from build123d import *

# Parameters (mm, degrees)
SKETCH1_W           = 237
SKETCH1_H           = 56
BOSS_EXTRUDE1_DEPTH = 4
SKETCH2_R           = 2
CUT_EXTRUDE1_DEPTH  = 5
SKETCH5_W           = 30
SKETCH5_H           = 4.1
BOSS_EXTRUDE2_DEPTH = 15
SKETCH6_W           = 4
SKETCH6_H           = 56
BOSS_EXTRUDE3_DEPTH = 25
FILLET1_START       = -119
FILLET1_DEPTH       = 238
FILLET3_R           = 4
FILLET4_R           = 4
FILLET5_R           = 4
FILLET6_R           = 4


with BuildPart() as part:
    # Sketch1 → Boss-Extrude1 (new body)
    with BuildSketch(Plane(origin=(0, 0, 0), x_dir=(1, 0, 0), z_dir=(0, 1, 0))):
        Rectangle(SKETCH1_W, SKETCH1_H)
    extrude(amount=BOSS_EXTRUDE1_DEPTH)

    # Sketch2 → Cut-Extrude1 (cut)
    with BuildSketch(Plane.XZ):
        with Locations(Location((108.5, 17.5, 0), (0, 0, 270))):
            Circle(SKETCH2_R)
        with Locations(Location((108.5, -17.5, 0), (0, 0, 270))):
            Circle(SKETCH2_R)
        with Locations(Location((-108.5, -17.5, 0), (0, 0, 270))):
            Circle(SKETCH2_R)
        with Locations(Location((-108.5, 17.5, 0), (0, 0, 270))):
            Circle(SKETCH2_R)
    extrude(amount=-CUT_EXTRUDE1_DEPTH, mode=Mode.SUBTRACT)

    # Sketch5 → Boss-Extrude2 (add)
    with BuildSketch(Plane(origin=(0, 4, 0), x_dir=(1, 0, 0), z_dir=(0, 1, 0))):
        with Locations((0, -25.95)):
            Rectangle(SKETCH5_W, SKETCH5_H)
        with Locations((25, 25.95)):
            Rectangle(SKETCH5_W, SKETCH5_H)
        with Locations((-25, 25.95)):
            Rectangle(SKETCH5_W, SKETCH5_H)
    extrude(amount=BOSS_EXTRUDE2_DEPTH)

    # Sketch6 → Boss-Extrude3 (add)
    with BuildSketch(Plane(origin=(0, 4, 0), x_dir=(1, 0, 0), z_dir=(0, 1, 0))):
        with Locations((-97.5, 0)):
            Rectangle(SKETCH6_W, SKETCH6_H)
        with Locations((97.5, 0)):
            Rectangle(SKETCH6_W, SKETCH6_H)
    extrude(amount=BOSS_EXTRUDE3_DEPTH)

    # Fillet1: read off the stored shape, not the designer's step
    # Fillet1 outline → Fillet1 (cut)
    with BuildSketch(Plane.YZ.offset(FILLET1_START)):
        with BuildLine():
            ThreePointArc((4, -28), (1.171572875, -26.828427125), (0, -24))
            Line((0, -24), (0, -28))
            Line((0, -28), (4, -28))
        make_face()
    extrude(amount=FILLET1_DEPTH, mode=Mode.SUBTRACT)

    # Fillet3
    fillet3_edges = [part.edges().sort_by_distance(p)[0] for p in [
        (0, 4, 23.9),
        (25, 4, -23.9),
        (-25, 4, -23.9),
        (-95.5, 4, 0),
        (95.5, 4, 0),
    ]]
    fillet(fillet3_edges, radius=FILLET3_R)

    # Fillet4
    # the kernel refuses this fillet: 4 mm, written as the material it takes off along each edge
    with BuildSketch(Plane(origin=(-118.5, 4, -38), x_dir=(0, -1, 0), z_dir=(0, 0, 1)), Plane(origin=(-99.5, 29, -38), x_dir=(0, -1, 0), z_dir=(0, 0, 1))) as fillet4_piece_1:
        with BuildLine():
            CenterArc((FILLET4_R, FILLET4_R), FILLET4_R, 180, 90)
            Line((0, FILLET4_R), (0, 0))
            Line((0, 0), (FILLET4_R, 0))
        make_face()
    extrude(amount=76, mode=Mode.SUBTRACT)
    with BuildSketch(Plane(origin=(118.5, 4, 38), x_dir=(-1, 0, 0), z_dir=(0, 0, -1)), Plane(origin=(99.5, 29, 38), x_dir=(-1, 0, 0), z_dir=(0, 0, -1))) as fillet4_piece_2:
        with BuildLine():
            CenterArc((FILLET4_R, -FILLET4_R), FILLET4_R, 90, 90)
            Line((0, -FILLET4_R), (0, 0))
            Line((0, 0), (FILLET4_R, 0))
        make_face()
    extrude(amount=76, mode=Mode.SUBTRACT)
    with BuildSketch(Plane(origin=(-99.5, 4, -28), x_dir=(1, 0, 0), z_dir=(0, 1, 0)), Plane(origin=(99.5, 4, 28), x_dir=(-1, 0, 0), z_dir=(0, 1, 0))) as fillet4_piece_3:
        with BuildLine():
            CenterArc((FILLET4_R, -FILLET4_R), FILLET4_R, 90, 90)
            Line((0, -FILLET4_R), (0, 0))
            Line((0, 0), (FILLET4_R, 0))
        make_face()
    extrude(amount=35, mode=Mode.SUBTRACT)
    with BuildSketch(Plane(origin=(-99.5, 4, 28), x_dir=(1, 0, 0), z_dir=(0, 1, 0)), Plane(origin=(99.5, 4, -28), x_dir=(-1, 0, 0), z_dir=(0, 1, 0))) as fillet4_piece_4:
        with BuildLine():
            CenterArc((FILLET4_R, FILLET4_R), FILLET4_R, 180, 90)
            Line((0, FILLET4_R), (0, 0))
            Line((0, 0), (FILLET4_R, 0))
        make_face()
    extrude(amount=35, mode=Mode.SUBTRACT)

    # Fillet5
    fillet5_edges = [part.edges().sort_by_distance(p)[0] for p in [
        (15, 11.5, 28),
        (-15, 11.5, 28),
        (0, 19, 28),
    ]]
    fillet(fillet5_edges, radius=FILLET5_R)

    # Fillet6
    fillet6_edges = [part.edges().sort_by_distance(p)[0] for p in [
        (25, 19, -28),
        (-25, 19, -28),
    ]]
    fillet(fillet6_edges, radius=FILLET6_R)


solid = part.part
Here's how the part is built. I have some questions about the finished solid (model axes, mm). A direction names the side the tool comes from. Round coordinates to 2 decimals unless told otherwise and drop trailing zeros. Order: outer loops, then holes, each group sorted by start corner. A loop starts at its lowest first (then second) coordinate and runs counter-clockwise, first axis right, second up. Notation, with made-up numbers: (48.25, 86.25) -> (105.25, 86.25) arc R31 ccw to (105.25, 118.25) -> close; hole circle Ø2 at (88, 42.25). An arc over 180 degrees is marked (long way). Use CSV: the item, a comma, the result in double quotes.
1. Thinking about a two-plate mould opening in X: for faces 1 (the face through (-117.297, 2.859, -0.392)), 2 (the face through (-24.79, 17.797, -26.859)), 3 (the face through (-1.659, 1.203, -26.859)), which applies, pulls with the +X half, pulls with the -X half, needs draft (parallel to the pull), parting line crosses it, or undercut?
Recorded:
face 1,"pulls with the -X half"
face 2,"undercut"
face 3,"needs draft"
2. I'm going to push flat-ended pins straight in: P1, Ø9, axis at x = -2, y = 16, coming from the -Z side; P2, Ø17, axis at y = 10, z = -3.5, coming from the -X side; P3, Ø5, axis at y = 12, z = 12.5, coming from the -X side; P4, Ø5, axis at x = -58, z = -4.5, coming from the -Y side. Where does each tip first touch, or does it pass through?
Recorded:
P1,"stops at z = 23.9"
P2,"stops at x = -118.21"
P3,"stops at x = -99.5"
P4,"stops at y = 0"
3. Which directions (+Z, -Z, +X, -X, +Y, -Y) give clear straight access to the entire face, cutting with the end or side of a thin tool? Please do faces 4 (the face through (10, 10, -26)), 5 (the face through (40, 10, -26)), 6 (the face through (-15, 6.5, 23.8)), 7 (the face through (-98.297, 16.325, -26.859)), 8 (the face through (-98.359, 16.325, 26.797)).
Recorded:
face 4,"-Z, +Y"
face 5,"+Z, -Z, +Y"
face 6,"+Z, +Y"
face 7,"-Z, -X, +Y"
face 8,"+Z, -X, +Y"
4. I want a section at C-C on x = -28. List the corners of the cut face in (y, z) for me.
Recorded:
outline,"(0, -24) arc R4 ccw to (4, -28) -> (15, -28) arc R4 ccw to (19, -24) -> (19, -23.9) -> (8, -23.9) arc R4 cw to (4, -19.9) -> (4, 28) -> (0, 28) -> close"
5. I want a section at D-D on z = -4.5. List the corners of the cut face in (x, y) for me.
Recorded:
outline,"(-118.5, 0) -> (118.5, 0) arc R4 ccw to (114.5, 4) -> (99.5, 4) -> (99.5, 25) arc R4 ccw to (95.5, 29) -> (95.5, 8) arc R4 cw to (91.5, 4) -> (-91.5, 4) arc R4 cw to (-95.5, 8) -> (-95.5, 29) arc R4 ccw to (-99.5, 25) -> (-99.5, 4) -> (-114.5, 4) arc R4 ccw to start"
6. I want a section at B-B on z = -17.5. List the corners of the cut face in (x, y) for me, and give its area (3 significant figures).
Recorded:
outline,"(-118.5, 0) -> (-110.5, 0) -> (-110.5, 4) -> (-114.5, 4) arc R4 ccw to start; (-106.5, 0) -> (106.5, 0) -> (106.5, 4) -> (99.5, 4) -> (99.5, 25) arc R4 ccw to (95.5, 29) -> (95.5, 8) arc R4 cw to (91.5, 4) -> (-91.5, 4) arc R4 cw to (-95.5, 8) -> (-95.5, 29) arc R4 ccw to (-99.5, 25) -> (-99.5, 4) -> (-106.5, 4) -> close; (110.5, 0) -> (118.5, 0) arc R4 ccw to (114.5, 4) -> (110.5, 4) -> close"
area,"1,110 mm2"
7. I want a section at A-A on y = 11.5. List the corners of the cut face in (x, z) for me, and give its area (3 significant figures).
Recorded:
outline,"(-99.5, -24) arc R4 ccw to (-95.5, -28) -> (-95.5, 28) arc R4 ccw to (-99.5, 24) -> close; (-40, -28) -> (-10, -28) -> (-10, -23.9) -> (-40, -23.9) -> close; (-15, 23.9) -> (15, 23.9) -> (15, 24) arc R4 ccw to (11, 28) -> (-11, 28) arc R4 ccw to (-15, 24) -> close; (10, -28) -> (40, -28) -> (40, -23.9) -> (10, -23.9) -> close; (95.5, -28) arc R4 ccw to (99.5, -24) -> (99.5, 24) arc R4 ccw to (95.5, 28) -> close"
area,"796 mm2"
8. I need wall thicknesses on line 1 along X through (y, z) = (14, -24); line 2 along X through (y, z) = (8.75, 15.5); line 3 along Y through (x, z) = (-23, 13.5). Which ranges of each line are inside material? Lowest first, please.
Recorded:
line 1,"x = -99.5 to -95.5, -40 to -10, 10 to 40, 95.5 to 99.5"
line 2,"x = -99.5 to -95.5, 95.5 to 99.5"
line 3,"y = 0 to 4"
